Check sheet for the drawn part. Datum: minimum x, y, z corner. Units: mm. Give positions to 0.01 mm unless a question says otherwise; leave off trailing zeros. Loops run counter-clockwise (first coordinate to the right, second up) from the corner with the lowest first, then second, coordinate; pieces in that order, holes last. Notation, with made-up numbers: (-29, 41) - (1, 41) arc R24 cw to (1, 70) - close; hole circle Ø8 at (24.5, 32). An arc over 180 degrees is marked (long way). One line per item, written item: value. Start each with the question number.
1. Sectioned sample at A-A (z = 1.5). Record the cut outline in (x, y), plus the area to 3 significant figures.
2. Sectioned sample at C-C (x = 44). Record the cut outline in (y, z).
3. Scan lines: L1, parallel to X at y = 43, z = 4.25; L2, parallel to Y at x = 43.5, z = 4.5; L3, parallel to X at y = 275, z = 4. Record each from-to range of solid material in increasing order. Write a range as [from, to].
4. Gauge pin test, flat end, axial feed: pin 1 (3 mm diameter, centred on x = 36, z = 2.5, fed in from -Y). Record the tip position at first contact, or that the pin passes through.
5. Sectioned sample at B-B (y = 265). Record the cut outline in (x, z).
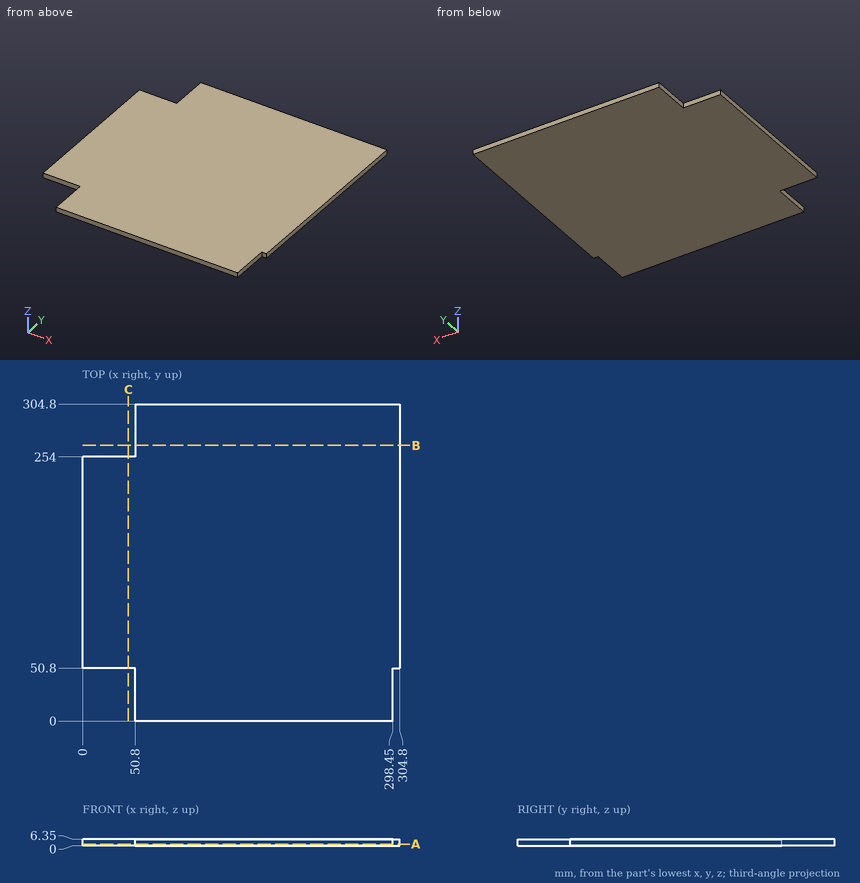
Results are:
1. outline: (0, 50.8) - (50.8, 50.8) - (50.8, 0) - (298.45, 0) - (298.45, 50.8) - (304.8, 50.8) - (304.8, 304.8) - (50.8, 304.8) - (50.8, 254) - (0, 254) - close
1. area: 87,400 mm^2
2. outline: (50.8, 0) - (254, 0) - (254, 6.35) - (50.8, 6.35) - close
3. L1: x = [50.8, 298.45]
3. L2: y = [50.8, 254]
3. L3: x = [50.8, 304.8]
4. pin 1: stops at y = 50.8
5. outline: (50.8, 0) - (304.8, 0) - (304.8, 6.35) - (50.8, 6.35) - close
